from build123d import *

# Parameters (mm, degrees)
F0_R             = 30
F0_R_2           = 6
F1_DEPTH         = 4
F2_DEPTH         = 6
F3_R             = 1.5
F4_DEPTH         = 12.5
F5_W             = 4.6
F5_H             = 3
F6_DEPTH         = 9.4
F9_R             = 7.5
F10_DEPTH        = 25
F10_COPIES_COUNT = 6


# Not quite as in the source:
# - a pattern or mirror of a feature is missing from the dataset's text; its kind, count and spacing are read off the source's solid


with BuildPart() as f1:
    # F0 (on Top) → F1 (new body)
    with BuildSketch(Plane.XY):
        Circle(F0_R)
        Circle(F0_R_2, mode=Mode.SUBTRACT)
        Circle(F0_R_2)
    extrude(amount=-F1_DEPTH)

    # F0 (on Top) → F2 (join)
    with BuildSketch(Plane.XY):
        Circle(F0_R_2)
    extrude(amount=F2_DEPTH)

    # F3 (on Front) → F4 (cut, symmetric)
    with BuildSketch(Plane.XZ):
        with Locations((0, 3)):
            Circle(F3_R)
    extrude(amount=F4_DEPTH, both=True, mode=Mode.SUBTRACT)

    # F5 (on face) → F6 (cut)
    with BuildSketch(Plane.XY.offset(6)):
        Rectangle(F5_W, F5_H)
        with BuildLine():
            ThreePointArc((-2.3, 1.5), (-2.7459060435, 0), (-2.3, -1.5))
            Line((-2.3, -1.5), (-2.3, 1.5))
        make_face()
        with BuildLine():
            Line((2.3, 1.5), (2.3, -1.5))
            ThreePointArc((2.3, -1.5), (2.745183651, 0), (2.3, 1.5))
        make_face()
    extrude(amount=-F6_DEPTH, mode=Mode.SUBTRACT)

    # F7 (on Front) → F8 (revolve, cut)
    with BuildSketch(Plane.XZ):
        Polygon((30, -3.4142135624), (30, -0.5857864376), (28.5857864376, -2), align=None)
    revolve(axis=Axis((0, 0, 0.7614716887), (0, 0, -1)), mode=Mode.SUBTRACT)

    # F9 (on face) → F10 (cut)
    with BuildSketch(Plane.XY):
        with Locations((0, 18.75)):
            Circle(F9_R)
    f10 = extrude(amount=-F10_DEPTH, mode=Mode.SUBTRACT)

    # F10_copies: F10 ×6 about axis
    f10_copies_axis = Axis((0, 0, 0), (0, 0, 1))
    for i in range(1, F10_COPIES_COUNT):
        add(f10.rotate(f10_copies_axis, i * 360 / F10_COPIES_COUNT), mode=Mode.SUBTRACT)


solid = f1.part
The listing builds one solid part. Answer for the finished solid, in the listing's coordinates (mm). A direction names the side the tool comes from. Round coordinates to 2 decimals unless told otherwise and drop trailing zeros. Use one line per item in the form item = value. Start each with the question number.
Item 1: Determine the mould class of faces 1 (the cylindrical face through (-2.746, 0.022, 1.366)), 2 (the cylindrical face through (-0.325, 3.721, 1.536)), 3 (the flat face through (6.2, 0.4, 0)) for opening direction Z: +Z half, -Z half, draft (parallel to the pull), parting line (faces both ways), or undercut.
Item 2: Flat-ended cylindrical pins translate along their axes: pin 1 Ø17 at (x, y) = (-16.24, 9.38) entering from +Z; pin 2 Ø1.4 at (x, z) = (0, 3) entering from +Y; pin 3 Ø1.5 at (x, y) = (0.5, 0) entering from +Z; pin 4 Ø4 at (x, z) = (0, 3) entering from -Y. Find the tip coordinate at first contact, or state that the pin passes through.
Item 3: Find the intervals of material crossed by line 1 (Y direction, x = -22.5, z = -0.5); line 2 (Y direction, x = -14.5, z = -2.25); line 3 (X direction, y = -3.5, z = -0.25), in increasing order. Write a range as [from, to].
Item 4: A cutting plane is placed at A-A (x = 0). Give the number of separate pieces and of enclosed holes in the cut face, plus the area to 3 significant figures.
Item 5: A tool of negligible diameter and unlimited length cuts with its end or side. For faces 4 (the cylindrical face through (-0.976, 26.186, -1.972)), 5 (the cylindrical face through (5.54, -2.3, 2.96)), from which of +Z, -Z, +X, -X, +Y, -Y can it reach the whole face along a straight path? Write none if from no direction.
The answers:
q1.face_1 = draft
q1.face_2 = undercut
q1.face_3 = +Z half
q2.pin_1 = 0
q2.pin_2 = through
q2.pin_3 = -3.4
q2.pin_4 = -6
q3.line_1 = [-19.84, -13.5], [-5.25, 5.25], [13.5, 19.84]
q3.line_2 = [-24.92, -16.67], [-2.08, 2.08], [16.67, 24.92]
q3.line_3 = [-29.8, -20.9], [-11.58, 11.58], [20.9, 29.8]
q4.separate_pieces = 5
q4.enclosed_holes = 0
q4.area = 133 mm^2
q5.face_4 = +Z, -Z
q5.face_5 = +Z
